from build123d import *

# Parameters (mm, degrees)
SKETCH1_W          = 4.5
SKETCH1_H          = 28.11709914
CUT_EXTRUDE1_DEPTH = 7
CUT_EXTRUDE2_DEPTH = 7
CHAMFER1_SIZE      = 0.5


with BuildPart() as part:
    # Sketch1 → Revolve-Thin1 (revolve)
    with BuildSketch(Plane(origin=(0, 0, 0), x_dir=(1, 0, 0), z_dir=(0, 1, 0))):
        with Locations((2.25, 31.55854957)):
            Rectangle(SKETCH1_W, SKETCH1_H)
    revolve(axis=Axis((0, 0, 0), (0, 0, -1)))

    # Sketch2 → Cut-Extrude1 (cut)
    with BuildSketch(Plane.XY.offset(-17.5)):
        Polygon((1.610807251, 2.79), (-1.610807251, 2.79), (-3.221614502, 0), (-1.610807251, -2.79), (1.610807251, -2.79), (3.221614502, 0), align=None)
    extrude(amount=-CUT_EXTRUDE1_DEPTH, mode=Mode.SUBTRACT)

    # Sketch3 → Cut-Extrude2 (cut)
    with BuildSketch(Plane(origin=(0, 0, -45.61709914), x_dir=(-1, 0, 0), z_dir=(0, 0, -1))):
        Polygon((1.610807251, 2.79), (-1.610807251, 2.79), (-3.221614502, 0), (-1.610807251, -2.79), (1.610807251, -2.79), (3.221614502, 0), align=None)
    extrude(amount=-CUT_EXTRUDE2_DEPTH, mode=Mode.SUBTRACT)

    # Chamfer1
    chamfer1_edges = [part.edges().sort_by_distance(p)[0] for p in [
        (2.416210877, 1.395, -17.5),
        (0, 2.79, -17.5),
        (-2.416210877, 1.395, -17.5),
        (-2.416210877, -1.395, -17.5),
        (0, -2.79, -17.5),
        (2.416210877, -1.395, -17.5),
        (-2.416210877, 1.395, -45.61709914),
        (0, 2.79, -45.61709914),
        (2.416210877, 1.395, -45.61709914),
        (2.416210877, -1.395, -45.61709914),
        (0, -2.79, -45.61709914),
        (-2.416210877, -1.395, -45.61709914),
    ]]
    chamfer(chamfer1_edges, length=CHAMFER1_SIZE)


solid = part.part
Could you check a few things on this model? Use its own coordinates, in mm. A direction names the side the tool comes from. Coordinates: 2 decimals unless noted, no trailing zeros. Loops run counter-clockwise (first coordinate to the right, second up) from the corner with the lowest first, then second, coordinate; pieces in that order, holes last.
1. Imagine slicing it at C-C (z = -32.5). Please give me the cut outline in (x, y), and give its area (3 significant figures).
2. For P1, Ø5, axis at y = 3, z = -21.5, coming from the +X side; P2, Ø3, axis at x = -0.5, y = -1.5, coming from the -Z side; P3, Ø3, axis at x = 2.5, z = -28, coming from the +Y side, each with a flat end and sliding along its axis, tell me the tip position at first contact or that it passes through.
3. Imagine slicing it at B-B (x = 0). Please give me the cut outline in (y, z), and give its area (3 significant figures).
4. We'd pull the mould along X, two halves only. Please class faces 1 (the face through (-0.59, -4.46, -31.76)), 2 (the face through (3, 2, -17.5)), 3 (the face through (0, 0, -38.617)): released by +X, released by -X, zero draft, split by the parting line, or undercut.
5. Imagine slicing it at A-A (z = -43). Please give me the cut outline in (x, y).
6. I need wall thicknesses on L1, parallel to Z at x = -0.75, y = -1; L2, parallel to X at y = -0.5, z = -18.75; L3, parallel to X at y = -2.5, z = -40. Which ranges of each line are inside material? Lowest first, please.
7. Imagine slicing it at D-D (y = -3.75). Please give me the cut outline in (x, z), and give its area (3 significant figures).
8. For faces 4 (the face through (2.405, 1.415, -41.913)), 5 (the face through (2.643, 1.495, -17.754)), which set-ups out of +Z, -Z, +X, -X, +Y, -Y let a thin tool reach every point of the face, with its end or its side?
Computed values:
1. outline: circle Ø9 at (0, 0)
1. area: 63.6 mm2
2. P1: stops at x = 4.47
2. P2: stops at z = -45.33
2. P3: stops at y = 4.39
3. outline: (-4.5, -45.62) - (-3.29, -45.62) - (-2.79, -45.12) - (-2.79, -38.62) - (2.79, -38.62) - (2.79, -45.12) - (3.29, -45.62) - (4.5, -45.62) - (4.5, -17.5) - (3.29, -17.5) - (2.79, -18) - (2.79, -24.5) - (-2.79, -24.5) - (-2.79, -18) - (-3.29, -17.5) - (-4.5, -17.5) - close
3. area: 174 mm2
4. face 1: split by the parting line
4. face 2: zero draft
4. face 3: undercut
5. outline: circle Ø9 at (0, 0); hole (-3.22, 0) - (-1.61, -2.79) - (1.61, -2.79) - (3.22, 0) - (1.61, 2.79) - (-1.61, 2.79) - close
6. L1: z = -38.62 to -24.5
6. L2: x = -4.47 to -2.93, 2.93 to 4.47
6. L3: x = -3.74 to -1.78, 1.78 to 3.74
7. outline: (-2.49, -45.62) - (2.49, -45.62) - (2.49, -17.5) - (-2.49, -17.5) - close
7. area: 140 mm2
8. face 4: -Z
8. face 5: +Z
